```python
from build123d import *

# Parameters (mm, degrees)
SKETCH1_R           = 15
SKETCH1_R_2         = 12.5
BOSS_EXTRUDE2_DEPTH = 30
SKETCH3_R           = 15
SKETCH3_R_2         = 12.5
BOSS_EXTRUDE3_DEPTH = 30
SKETCH4_R           = 12.5
CUT_EXTRUDE1_DEPTH  = 18


with BuildPart() as part:
    # Sketch1 → Boss-Extrude2 (new body)
    with BuildSketch(Plane.XY):
        with BuildLine():
            ThreePointArc((15, 0), (0, -15), (-15, 0))
            Line((-15, 0), (-15, -15))
            Line((-15, -15), (-15, -18))
            Line((-15, -18), (15, -18))
            Line((15, -18), (15, 0))
        make_face()
        Circle(SKETCH1_R)
        Circle(SKETCH1_R_2, mode=Mode.SUBTRACT)
    extrude(amount=BOSS_EXTRUDE2_DEPTH)

    # Sketch3 → Boss-Extrude3 (add)
    with BuildSketch(Plane.XZ.offset(18)):
        with Locations((0, 15)):
            Circle(SKETCH3_R)
        with Locations((0, 15)):
            Circle(SKETCH3_R_2, mode=Mode.SUBTRACT)
    extrude(amount=BOSS_EXTRUDE3_DEPTH)

    # Sketch4 → Cut-Extrude1 (cut)
    with BuildSketch(Plane.XZ.offset(18)):
        with Locations((0, 15)):
            Circle(SKETCH4_R)
    extrude(amount=-CUT_EXTRUDE1_DEPTH, mode=Mode.SUBTRACT)


solid = part.part
```
CAD build for the part. Positions are in the model's coordinates, mm. A direction names the side the tool comes from. Coordinates: 2 decimals unless noted, no trailing zeros. Order: outer loops, then holes, each group sorted by start corner. A loop starts at its lowest first (then second) coordinate and runs counter-clockwise, first axis right, second up. Notation, with made-up numbers: (58.5, 30) -> (91.5, 30) arc R22 ccw to (91.5, 66) -> close; hole circle Ø6 at (27, 89). An arc over 180 degrees is marked (long way). Use one line per item in the form item = value. Start each with the question number.
1) Band-saw the part on D-D on y = -19.5. Give the cut face in (x, z).
2) Band-saw the part on A-A on x = 8.5. Give the cut face in (y, z).
3) Band-saw the part on B-B on y = -1.5. Give the cut face in (x, z), then the cut area to 3 significant figures.
4) Pull direction Y, two halves, no side cores. Call faces 5 (the flat face through (3.1, -12.3, 30)), 6 (the flat face through (-12, -18, 26)), 7 (the cylindrical face through (-1.627, 12.394, 14.79)): +Y half, -Y half, draft (parallel to the pull), parting line (faces both ways), or undercut.
5) Drill centre lines: L1, parallel to Z at x = 0, y = -13.25; L2, parallel to Y at x = -0.5, z = 2.25; L3, parallel to Y at x = 0, z = 20. Where is each one in solid material? Low to high. Write a range as [from, to].
6) Drop flat-ended pins along their axis: pin 1 (7.5 mm diameter, centred on x = 10.5, z = 10, fed in from -Y); pin 2 (2 mm diameter, centred on x = -6.5, z = 25.5, fed in from +Y); pin 3 (6 mm diameter, centred on x = -9.5, y = -35.5, fed in from +Z); pin 4 (1.5 mm diameter, centred on y = -20, z = 3.5, fed in from +X). Give the stop position or say it passes through.
7) Tool access for faces 1 (the flat face through (11, -18, 3)), 2 (the flat face through (12, -18, 27)), 3 (the flat face through (-12, -18, 4)), 4 (the cylindrical face through (-3.252, -32.79, 0.357)): list every direction of +Z, -Z, +X, -X, +Y, -Y with a clear straight run to the whole face (end or side of a thin tool).
8) Band-saw the part on C-C on z = 18.25. Give the cut face in (x, y).
Entries:
q1.outline = circle Ø30 at (0, 15); hole circle Ø25 at (0, 15)
q2.outline = (-48, 2.64) -> (-18, 2.64) -> (-18, 0) -> (-9.17, 0) -> (-9.17, 5.83) -> (-48, 5.83) -> close; (-48, 24.17) -> (-9.17, 24.17) -> (-9.17, 30) -> (-18, 30) -> (-18, 27.36) -> (-48, 27.36) -> close; (9.17, 0) -> (12.36, 0) -> (12.36, 30) -> (9.17, 30) -> close
q3.outline = (-15, 0) -> (-12.41, 0) -> (-12.41, 13.5) arc R12.5 cw to (-12.41, 16.5) -> (-12.41, 30) -> (-15, 30) -> close; (12.41, 0) -> (15, 0) -> (15, 30) -> (12.41, 30) -> (12.41, 16.5) arc R12.5 cw to (12.41, 13.5) -> close
q3.area = 155 mm2
q4.face_5 = draft
q4.face_6 = -Y half
q4.face_7 = undercut
q5.L1 = [0, 2.5], [27.5, 30]
q5.L2 = [-48, -12.49], [12.49, 14.99]
q5.L3 = [12.5, 15]
q6.pin_1 = -48
q6.pin_2 = 13.96
q6.pin_3 = 28.52
q6.pin_4 = 10.46
q7.face_1 = -Z, +X, -Y
q7.face_2 = +Z, +X, -Y
q7.face_3 = -Z, -X, -Y
q7.face_4 = -Y
q8.outline = (-15, -18) -> (-14.64, -18) -> (-14.64, -48) -> (-12.07, -48) -> (-12.07, -3.25) arc R12.5 cw (long way) to (12.07, -3.25) -> (12.07, -48) -> (14.64, -48) -> (14.64, -18) -> (15, -18) -> (15, 0) arc R15 ccw to (-15, 0) -> close
